Model file for the job. Use its own axes, mm. A direction names the side the tool comes from. Coordinates: 2 decimals unless noted, no trailing zeros. Order: outer loops, then holes, each group sorted by start corner. A loop starts at its lowest first (then second) coordinate and runs counter-clockwise, first axis right, second up. Notation, with made-up numbers: (36, -1) -> (68, -1) arc R21 ccw to (68, 34) -> close; hole circle Ø6 at (3, -5.5). An arc over 180 degrees is marked (long way). Use CSV: the item, a comma, the result in double quotes. Start each with the question number.
(1) Tool access for faces 1 (the flat face through (2, -2, 0)), 2 (the cylindrical face through (-14.985, 0.66, -32.465)), 3 (the flat face through (0.1, 13.4, -35)): list every direction of +Z, -Z, +X, -X, +Y, -Y with a clear straight run to the whole face (end or side of a thin tool).
(2) Cut at A-A on z = -31. Write the cut outline in (x, y), plus the area to 3 significant figures.
(3) Cut at B-B on y = -18. Write the cut outline in (x, z).
(4) Pin check, flat tips, straight feed: pin 1 Ø2 at (x, y) = (0, 0.5) entering from +Z; pin 2 Ø12 at (y, z) = (-4.5, -5) entering from +X; pin 3 Ø15 at (x, y) = (3, 3.5) entering from +Z; pin 4 Ø10 at (x, y) = (-11, -10.5) entering from +Z. Stop position of each tip, or through.
(5) Probe L1, parallel to Y at x = 0, z = -6.25; L2, parallel to Z at x = -8.5, y = 11.5; L3, parallel to Y at x = 0, z = -3.75. List the from-to ranges inside material, lowest first.
(6) Cut at C-C on z = -41.5. Write the cut outline in (x, y), plus the area to 3 significant figures.
(7) Pull direction X, two halves, no side cores. Call faces 4 (the flat face through (3, 15, -40)), 5 (the cylindrical face through (-4.336, -19.524, -44.93)), 6 (the conical face through (-0.278, 2.117, -11.458)), 7 (the flat face through (0, 0, -12)): pulls with the +X half, pulls with the -X half, needs draft (parallel to the pull), parting line crosses it, or undercut.
```python
from build123d import *


with BuildPart() as f1:
    # F0 (on Front) → F1 (revolve)
    with BuildSketch(Plane.XZ):
        with BuildLine():
            Line((3.5, 0), (2.5, 0))
            Line((2.5, 0), (2.5, -10))
            Line((2.5, -10), (2, -12))
            Line((2, -12), (0, -12))
            Line((0, -12), (0, -50))
            Line((0, -50), (20, -50))
            Line((20, -50), (20, -40))
            Line((20, -40), (15, -40))
            Line((15, -40), (15, -37))
            Line((15, -37), (13, -37))
            Line((13, -37), (13, -35))
            Line((13, -35), (15, -35))
            Line((15, -35), (15, -30))
            Line((15, -30), (13, -30))
            Line((13, -30), (13, -27))
            Line((13, -27), (15, -27))
            Line((15, -27), (15, -20))
            ThreePointArc((15, -20), (7.9289321881, -17.0710678119), (5, -10))
            Line((5, -10), (5, -4))
            Line((5, -4), (3.5, 0))
        make_face()
    revolve(axis=Axis((0, 0, -25), (0, 0, 1)))


solid = f1.part
```
Outcome:
1,face 1,"+Z, +X, -X, +Y, -Y"
1,face 2,"+Z"
1,face 3,"none"
2,outline,"circle Ø30 at (0, 0)"
2,area,"707 mm2"
3,outline,"(-8.72, -50) -> (8.72, -50) -> (8.72, -40) -> (-8.72, -40) -> close"
4,pin 1,"z = -12"
4,pin 2,"x = 5"
4,pin 3,"z = 0"
4,pin 4,"z = -18.78"
5,L1,"-5 to -2.5, 2.5 to 5"
5,L2,"-50 to -37, -35 to -30, -27 to -19.98"
5,L3,"-4.91 to -2.5, 2.5 to 4.91"
6,outline,"circle Ø40 at (0, 0)"
6,area,"1,260 mm2"
7,face 4,"needs draft"
7,face 5,"parting line crosses it"
7,face 6,"undercut"
7,face 7,"undercut"
